from build123d import *

# Parameters (mm, degrees)
F0_W      = 558.8
F0_H      = 558.8
F1_DEPTH  = 12.7
F2_W      = 355.6
F2_H      = 12.7
F3_DEPTH  = 114.3
F4_W      = 330.2
F4_H      = 330.2
F5_DEPTH  = 25.4
F6_W      = 381
F6_H      = 381
F6_W_2    = 330.2
F6_H_2    = 330.2
F7_DEPTH  = 25.4
F8_W      = 76.2
F8_H      = 38.1
F9_DEPTH  = 2.54
F10_W     = 76.2
F10_H     = 2.54
F11_DEPTH = 2.54
F13_DEPTH = 2.54
F15_DEPTH = 2.54


with BuildPart() as f1:
    # F0 (on Top) → F1 (new body)
    with BuildSketch(Plane.XY):
        Rectangle(F0_W, F0_H)
    extrude(amount=F1_DEPTH)

    # F2 (on face) → F3 (join)
    with BuildSketch(Plane(origin=(0, 0, 0), x_dir=(1, 0, 0), z_dir=(0, 0, -1))):
        with Locations((0, 273.05)):
            Rectangle(F2_W, F2_H)
    extrude(amount=F3_DEPTH)

    # F4 (on face) → F5 (cut)
    with BuildSketch(Plane.XY.offset(12.7)):
        Rectangle(F4_W, F4_H)
    extrude(amount=-F5_DEPTH, mode=Mode.SUBTRACT)

    # F6 (on face) → F7 (join)
    with BuildSketch(Plane.XY.offset(12.7)):
        Rectangle(F6_W, F6_H)
        Rectangle(F6_W_2, F6_H_2, mode=Mode.SUBTRACT)
    extrude(amount=F7_DEPTH)

    # F8 (on face) → F9 (join)
    with BuildSketch(Plane.XY.offset(12.7)):
        with Locations((-152.4, 260.35)):
            Rectangle(F8_W, F8_H)
        with Locations((152.4, 260.35)):
            Rectangle(F8_W, F8_H)
    extrude(amount=F9_DEPTH)

    # F10 (on face) → F11 (join)
    with BuildSketch(Plane(origin=(0, 279.4, 0), x_dir=(-1, 0, 0), z_dir=(0, 1, 0))):
        with Locations((-152.4, 13.97)):
            Rectangle(F10_W, F10_H)
        with Locations((152.4, 13.97)):
            Rectangle(F10_W, F10_H)
    extrude(amount=F11_DEPTH)

    # F12 (on face) → F13 (cut)
    with BuildSketch(Plane.XY.offset(15.24)):
        with BuildLine():
            Line((-158.75, 266.7), (-152.4, 266.7))
            Line((-152.4, 266.7), (-146.05, 266.7))
            ThreePointArc((-146.05, 266.7), (-152.4, 273.05), (-158.75, 266.7))
        make_face()
        with BuildLine():
            ThreePointArc((-158.75, 266.7), (-156.8901280605, 262.2098719395), (-152.4, 260.35))
            Line((-152.4, 260.35), (-152.4, 266.7))
            Line((-152.4, 266.7), (-158.75, 266.7))
        make_face()
        with BuildLine():
            Line((-152.4, 266.7), (-152.4, 260.35))
            ThreePointArc((-152.4, 260.35), (-147.9098719395, 262.2098719395), (-146.05, 266.7))
            Line((-146.05, 266.7), (-152.4, 266.7))
        make_face()
        with BuildLine():
            ThreePointArc((-171.45, 260.35), (-177.8, 254), (-171.45, 247.65))
            Line((-171.45, 247.65), (-171.45, 260.35))
        make_face()
        with BuildLine():
            Line((-171.45, 260.35), (-171.45, 247.65))
            ThreePointArc((-171.45, 247.65), (-166.9598719395, 249.5098719395), (-165.1, 254))
            ThreePointArc((-165.1, 254), (-166.9598719395, 258.4901280605), (-171.45, 260.35))
        make_face()
        with BuildLine():
            ThreePointArc((-133.35, 260.35), (-139.7, 254), (-133.35, 247.65))
            Line((-133.35, 247.65), (-133.35, 260.35))
        make_face()
        with BuildLine():
            Line((-133.35, 260.35), (-133.35, 247.65))
            ThreePointArc((-133.35, 247.65), (-128.8598719395, 249.5098719395), (-127, 254))
            ThreePointArc((-127, 254), (-128.8598719395, 258.4901280605), (-133.35, 260.35))
        make_face()
    extrude(amount=-F13_DEPTH, mode=Mode.SUBTRACT)

    # F14 (on face) → F15 (cut)
    with BuildSketch(Plane.XY.offset(15.24)):
        with BuildLine():
            Line((146.05, 266.7), (152.4, 266.7))
            Line((152.4, 266.7), (158.75, 266.7))
            ThreePointArc((158.75, 266.7), (152.4, 273.05), (146.05, 266.7))
        make_face()
        with BuildLine():
            ThreePointArc((146.05, 266.7), (147.9098719395, 262.2098719395), (152.4, 260.35))
            Line((152.4, 260.35), (152.4, 266.7))
            Line((152.4, 266.7), (146.05, 266.7))
        make_face()
        with BuildLine():
            Line((152.4, 266.7), (152.4, 260.35))
            ThreePointArc((152.4, 260.35), (156.8901280605, 262.2098719395), (158.75, 266.7))
            Line((158.75, 266.7), (152.4, 266.7))
        make_face()
        with BuildLine():
            ThreePointArc((171.45, 260.35), (165.1, 254), (171.45, 247.65))
            Line((171.45, 247.65), (171.45, 260.35))
        make_face()
        with BuildLine():
            Line((171.45, 260.35), (171.45, 247.65))
            ThreePointArc((171.45, 247.65), (175.9401280605, 249.5098719395), (177.8, 254))
            ThreePointArc((177.8, 254), (175.9401280605, 258.4901280605), (171.45, 260.35))
        make_face()
        with BuildLine():
            Line((133.35, 260.35), (133.35, 247.65))
            ThreePointArc((133.35, 247.65), (137.8401280605, 249.5098719395), (139.7, 254))
            ThreePointArc((139.7, 254), (137.8401280605, 258.4901280605), (133.35, 260.35))
        make_face()
        with BuildLine():
            ThreePointArc((133.35, 260.35), (127, 254), (133.35, 247.65))
            Line((133.35, 247.65), (133.35, 260.35))
        make_face()
    extrude(amount=-F15_DEPTH, mode=Mode.SUBTRACT)


solid = f1.part
Work out the finished part from the listing and answer in its coordinate system (mm). A direction names the side the tool comes from. Coordinates: 2 decimals unless noted, no trailing zeros. Write each loop counter-clockwise with the first axis right and the second up, starting at its lowest first coordinate (ties: lowest second). Pieces come first, ordered by that corner, then holes. Notation, with made-up numbers: M 46,18 L 56,18 A27 cw 56,39 Z; hole C 49.25,46.5 d5. An arc over 180 degrees is marked long. Write item = value, one per line.
1. The part is cut by section A-A (y = -115). Determine the outline of the cut face in (x, z).
Solution:
outline = M -279.4,0 L -165.1,0 L -165.1,38.1 L -190.5,38.1 L -190.5,12.7 L -279.4,12.7 Z; M 165.1,0 L 279.4,0 L 279.4,12.7 L 190.5,12.7 L 190.5,38.1 L 165.1,38.1 Z
2. For faces 4 (the face through (-177.8, -273, -56)), 5 (the face through (153, 257, 15.24)), 6 (the face through (190.5, -3, 25)), 7 (the face through (133, 254, 12.7)), 8 (the face through (-4, 279.4, 6)), determine the directions among +Z, -Z, +X, -X, +Y, -Y from which every point of the face is accessible in a straight line to the end or side of a thin tool.
Solution:
face_4 = -Z, -X, +Y, -Y
face_5 = +Z, +X, -X, +Y
face_6 = +Z, +X, +Y, -Y
face_7 = +Z
face_8 = -Z, +X, -X, +Y
3. The part is cut by section C-C (x = -237). Determine the outline of the cut face in (y, z), then the cut area to 3 significant figures.
Solution:
outline = M -279.4,0 L 279.4,0 L 279.4,12.7 L -279.4,12.7 Z
area = 7,100 mm2
4. Determine the mould class of faces 1 (the face through (279.4, -4, 6)), 2 (the face through (-3, -190.5, 25)), 3 (the face through (-165.1, -2, 19)) for opening direction X: released by +X, released by -X, zero draft, split by the parting line, or undercut.
Solution:
face_1 = released by +X
face_2 = zero draft
face_3 = undercut
5. Straight lines are drawn through the part: line 1 (X direction, y = -57, z = 14.5); line 2 (X direction, y = -110.5, z = 7); line 3 (Z direction, x = 240, y = 234). For each, find the intervals that lie inside material, in ascending order. Write a range as from..to.
Solution:
line_1 = -190.5..-165.1, 165.1..190.5
line_2 = -279.4..-165.1, 165.1..279.4
line_3 = 0..12.7
6. The part is cut by section B-B (x = -1). Determine the outline of the cut face in (y, z), then the cut area to 3 significant figures.
Solution:
outline = M -279.4,-114.3 L -266.7,-114.3 L -266.7,0 L -165.1,0 L -165.1,38.1 L -190.5,38.1 L -190.5,12.7 L -279.4,12.7 Z; M 165.1,0 L 279.4,0 L 279.4,12.7 L 190.5,12.7 L 190.5,38.1 L 165.1,38.1 Z
area = 5,650 mm2
7. Flat-ended cylindrical pins translate along their axes: pin 1 (0.8 mm diameter, centred on y = 271.5, z = 14, fed in from +X); pin 2 (14 mm diameter, centred on x = 133, y = 254, fed in from +Z); pin 3 (4 mm diameter, centred on x = -168.5, y = 256, fed in from +Z); pin 4 (3 mm diameter, centred on x = -134.5, z = 14, fed in from -Y). Find the tip coordinate at first contact, or state that the pin passes through.
Solution:
pin_1 = 190.5
pin_2 = 15.24
pin_3 = 12.7
pin_4 = -279.4
